Part model, mm, in its own coordinate system. A direction names the side the tool comes from. Give positions to 0.01 mm unless a question says otherwise; leave off trailing zeros. Write each loop counter-clockwise with the first axis right and the second up, starting at its lowest first coordinate (ties: lowest second). Pieces come first, ordered by that corner, then holes. Notation, with made-up numbers: M 76.25,-33.75 L 84.25,-33.75 A27 ccw 84.25,-8.75 Z; hole C 42.5,27.25 d2. An arc over 180 degrees is marked long. Use a Markdown table: item, result.
```python
from build123d import *

# Parameters (mm, degrees)
F1_DEPTH = 457.2
F2_R     = 25.4
F3_T     = -1.5875


with BuildPart() as f1:
    # F0 (on Top) → F1 (new body)
    with BuildSketch(Plane.XY):
        Polygon((76.2, -101.6), (76.2, 177.8), (-76.2, 177.8), (-76.2, -101.6), (0, -177.8), align=None)
    extrude(amount=F1_DEPTH)

    # F2
    f2_edges = [f1.edges().sort_by_distance(p)[0] for p in [
        (0, -177.8, 228.6),
        (76.2, -101.6, 228.6),
        (-76.2, -101.6, 228.6),
    ]]
    fillet(f2_edges, radius=F2_R)

    # F3
    f3_openings = [f1.faces().sort_by_distance(p)[0] for p in [
        (0, 18.896629, 0),
    ]]
    offset(amount=F3_T, openings=f3_openings)


solid = f1.part
```
1. Tool access for faces 1 (the cylindrical face through (72.85, -100.07, 231)), 2 (the flat face through (43, -134.8, 225.4)): list every direction of +Z, -Z, +X, -X, +Y, -Y with a clear straight run to the whole face (end or side of a thin tool).
Findings below:
| item | result |
|---|---|
| face 1 | -Z |
| face 2 | +Z, -Z, +X, -Y |
2. Drill centre lines: L1, parallel to X at y = -30.5, z = 422; L2, parallel to Y at x = -0.5, z = 391; L3, parallel to Z at x = 25.5, y = 43.5. Where is each one in solid material? Low to high.
Findings below:
| item | result |
|---|---|
| L1 | -76.2 to -74.61, 74.61 to 76.2 |
| L2 | -167.27 to -165.69, 176.21 to 177.8 |
| L3 | 455.61 to 457.2 |
3. Cut at C-C, the plane x = 23.5. Give the cut face in (y, z).
Findings below:
| item | result |
|---|---|
| outline | M -154.3,0 L -152.05,0 L -152.05,455.61 L 176.21,455.61 L 176.21,0 L 177.8,0 L 177.8,457.2 L -154.3,457.2 Z |
4. Cut at B-B, the plane y = -62. Give the cut face in (x, z).
Findings below:
| item | result |
|---|---|
| outline | M -76.2,0 L -74.61,0 L -74.61,455.61 L 74.61,455.61 L 74.61,0 L 76.2,0 L 76.2,457.2 L -76.2,457.2 Z |
5. Drop flat-ended pins along their axis: P1, Ø2, axis at x = -37, y = 129, coming from the -Z side; P2, Ø4, axis at x = 27.5, z = 345.5, coming from the -Y side; P3, Ø4, axis at y = -122.5, z = 389, coming from the -X side. Give the stop position or say it passes through.
Findings below:
| item | result |
|---|---|
| P1 | z = 455.61 |
| P2 | y = -152.3 |
| P3 | x = -57.3 |
6. Cut at A-A, the plane z = 418. Give the cut face in (x, y) (1 decimal), then the cut area to 3 significant figures.
Findings below:
| item | result |
|---|---|
| outline | M -76.2,-91.1 A25.4 ccw -68.8,-109 L -18,-159.8 A25.4 ccw 18,-159.8 L 68.8,-109 A25.4 ccw 76.2,-91.1 L 76.2,177.8 L -76.2,177.8 Z; hole M -74.6,-91.1 A23.8 ccw -67.6,-107.9 L -16.8,-158.7 A23.8 ccw 16.8,-158.7 L 67.6,-107.9 A23.8 ccw 74.6,-91.1 L 74.6,176.2 L -74.6,176.2 Z |
| area | 1,440 mm2 |
7. Two-plate mould, pull along Y, no slides. Class faces 3 (the cylindrical face through (74.32, -100.67, 231.8)), 4 (the flat face through (-76.2, 45, 225)), 5 (the flat face through (74.612, 41, 225)): released by +Y, released by -Y, zero draft, split by the parting line, or undercut.
Findings below:
| item | result |
|---|---|
| face 3 | released by -Y |
| face 4 | zero draft |
| face 5 | undercut |
